Work out the finished part from the listing and answer in its coordinate system (mm). A direction names the side the tool comes from. Round coordinates to 2 decimals unless told otherwise and drop trailing zeros. Write each loop counter-clockwise with the first axis right and the second up, starting at its lowest first coordinate (ties: lowest second). Pieces come first, ordered by that corner, then holes. Notation, with made-up numbers: (-37, -3.75) - (-26, -3.75) arc R19 cw to (-26, 14.25) - close; hole circle Ø6 at (71.25, 70.25). An arc over 180 degrees is marked (long way). Answer as a JSON object with one key per item and string values.
```python
from build123d import *

# Parameters (mm, degrees)
F0_R     = 56.515
F1_DEPTH = 101.6
F2_R     = 52.07
F3_DEPTH = 95.25
F4_R     = 63.5
F5_DEPTH = 3.175
F6_R     = 52.07
F7_DEPTH = 12.7
F8_R     = 7.62
F9_R     = 2.54
F10_R    = 2.54


# Not quite as in the source:
# - a fillet or chamfer that OpenCascade refuses, or shapes differently, is made with other operations: its cross-section is extruded or revolved along the edge and cut away or added


with BuildPart() as f1:
    # F0 (on Top) → F1 (new body)
    with BuildSketch(Plane.XY):
        Circle(F0_R)
    extrude(amount=F1_DEPTH)

    # F2 (on Top) → F3 (cut)
    with BuildSketch(Plane.XY):
        Circle(F2_R)
    extrude(amount=F3_DEPTH, mode=Mode.SUBTRACT)

    # F4 (on face) → F5 (join)
    with BuildSketch(Plane(origin=(0, 0, 0), x_dir=(1, 0, 0), z_dir=(0, 0, -1))):
        Circle(F4_R)
    extrude(amount=F5_DEPTH)

    # F6 (on Top) → F7 (cut)
    with BuildSketch(Plane.XY):
        Circle(F6_R)
    extrude(amount=-F7_DEPTH, mode=Mode.SUBTRACT)

    # F8
    f8_edges = [f1.edges().sort_by_distance(p)[0] for p in [
        (-56.515, 0, 101.6),
    ]]
    fillet(f8_edges, radius=F8_R)

    # F9
    f9_edges = [f1.edges().sort_by_distance(p)[0] for p in [
        (-52.07, 0, -3.175),
    ]]
    fillet(f9_edges, radius=F9_R)

    # F10
    f10_edges = [f1.edges().sort_by_distance(p)[0] for p in [
        (-63.5, 0, 0),
    ]]
    fillet(f10_edges, radius=F10_R)

    # F11: fillet of radius 2.54 on 1 edges, made by hand

    # F11_s1 → F11_t2 (revolve, cut)
    with BuildSketch(Plane.XZ):
        with BuildLine():
            ThreePointArc((63.5, -2.54), (62.7179735296, -3.0109524406), (61.8199479175, -3.175))
            Line((61.8199479175, -3.175), (63.5, -3.175))
            Line((63.5, -3.175), (63.5, -2.54))
        make_face()
    revolve(axis=Axis((0, 0, -3.175), (0, 0, -1)), mode=Mode.SUBTRACT)


solid = f1.part
```
Item 1: Consider line 1 along Y through (x, z) = (0, 37) (3 decimals); line 2 along Z through (x, y) = (19, 16); line 3 along Y through (x, z) = (21, 54.5). Determine where each line is inside the solid, lowest interval first.
Results found:
{"line 1": "-56.515 to -52.07, 52.07 to 56.515", "line 2": "95.25 to 101.6", "line 3": "-52.47 to -47.65, 47.65 to 52.47"}
Item 2: Determine the mould class of faces 1 (the flat face through (-1, 1, 95.25)), 2 (the flat face through (0, 55, -3.175)), 3 (the cylindrical face through (-44.848, -34.388, 46.332)) for opening direction X: pulls with the +X half, pulls with the -X half, needs draft (parallel to the pull), parting line crosses it, or undercut.
Results found:
{"face 1": "undercut", "face 2": "needs draft", "face 3": "parting line crosses it"}
Item 3: A cutting plane is placed at B-B (z = 55). Write down the section's boundary in (x, y) (3 decimals), and give its area (3 significant figures).
Results found:
{"outline": "circle Ø113.03 at (0, 0); hole circle Ø104.14 at (0, 0)", "area": "1,520 mm²"}
Item 4: For faces 4 (the flat face through (-1, 1, 101.6)), 5 (the flat face through (54, 18, 0)), determine the directions among +Z, -Z, +X, -X, +Y, -Y from which every point of the face is accessible in a straight line to the end or side of a thin tool.
Results found:
{"face 4": "+Z, +X, -X, +Y, -Y", "face 5": "+Z"}
Item 5: A cutting plane is placed at A-A (y = 0). Write down the section's boundary in (x, z) (3 decimals).
Results found:
{"outline": "(-63.5, -2.54) arc R2.54 ccw to (-61.82, -3.175) - (-54.61, -3.175) arc R2.54 ccw to (-52.07, -0.635) - (-52.07, 95.25) - (52.07, 95.25) - (52.07, -0.635) arc R2.54 ccw to (54.61, -3.175) - (61.82, -3.175) arc R2.54 ccw to (63.5, -2.54) arc R2.54 ccw to (60.96, 0) - (56.515, 0) - (56.515, 93.98) arc R7.62 ccw to (48.895, 101.6) - (-48.895, 101.6) arc R7.62 ccw to (-56.515, 93.98) - (-56.515, 0) - (-60.96, 0) arc R2.54 ccw to start"}
Item 6: Each of these flat-tipped pins is pushed along its axis until it touches: P1, Ø5, axis at y = 28.5, z = 29.5, coming from the -X side; P2, Ø3, axis at y = 11.5, z = 16, coming from the -X side; P3, Ø2, axis at y = 42, z = 30.5, coming from the -X side. Where does it stop, or does it pass through?
Results found:
{"P1": "x = -50.18", "P2": "x = -55.62", "P3": "x = -38.9"}
